from build123d import *

# Parameters (mm, degrees)
SKETCH1_R           = 2.286
BOSS_EXTRUDE1_DEPTH = 12.7
SKETCH5_R           = 2.286
CUT_EXTRUDE3_DEPTH  = 12.7
FILLET1_R           = 4.87
FILLET2_R           = 4.87
SKETCH7_W           = 50.304618045
SKETCH7_H           = 38.1
CUT_EXTRUDE4_DEPTH  = 6.35


with BuildPart() as part:
    # Sketch1 → Boss-Extrude1 (new body)
    with BuildSketch(Plane(origin=(0, 0, 0), x_dir=(1, 0, 0), z_dir=(0, 1, 0))):
        with BuildLine():
            Line((-291.755501553, 191.396492393), (-280.151228022, 178.973093671))
            ThreePointArc((-280.151228022, 178.973093671), (-270.685286175, 182.170263236), (-266.850883508, 191.396492393))
            Line((-266.850883508, 191.396492393), (-254.150883508, 191.396492393))
            Line((-254.150883508, 191.396492393), (-254.150883508, 127.896492393))
            Line((-254.150883508, 127.896492393), (-304.455501553, 127.896492393))
            Line((-304.455501553, 127.896492393), (-304.455501553, 191.396492393))
            Line((-304.455501553, 191.396492393), (-291.755501553, 191.396492393))
        make_face()
        with Locations(Location((-297.746130931, 134.246492393, 0), (0, 0, 270))):
            Circle(SKETCH1_R, mode=Mode.SUBTRACT)
        with Locations(Location((-278.990383135, 134.246492393, 0), (0, 0, 270))):
            Circle(SKETCH1_R, mode=Mode.SUBTRACT)
        with Locations(Location((-260.86025413, 134.246492393, 0), (0, 0, 270))):
            Circle(SKETCH1_R, mode=Mode.SUBTRACT)
    extrude(amount=BOSS_EXTRUDE1_DEPTH)

    # Sketch5 → Cut-Extrude3 (cut)
    with BuildSketch(Plane(origin=(0, 0, -191.396492393), x_dir=(-1, 0, 0), z_dir=(0, 0, -1))):
        with Locations((260.500883508, 6.35)):
            Circle(SKETCH5_R)
        with Locations((298.105501553, 6.35)):
            Circle(SKETCH5_R)
    extrude(amount=-CUT_EXTRUDE3_DEPTH, mode=Mode.SUBTRACT)

    # Fillet1
    fillet1_edges = [part.edges().sort_by_distance(p)[0] for p in [
        (-304.455501553, 6.35, -127.896492393),
    ]]
    fillet(fillet1_edges, radius=FILLET1_R)

    # Fillet2
    fillet2_edges = [part.edges().sort_by_distance(p)[0] for p in [
        (-254.150883508, 6.35, -127.896492393),
    ]]
    fillet(fillet2_edges, radius=FILLET2_R)

    # Sketch7 → Cut-Extrude4 (cut)
    with BuildSketch(Plane(origin=(0, 12.7, 0), x_dir=(1, 0, 0), z_dir=(0, 1, 0))):
        with Locations((-279.303192531, 146.946492393)):
            Rectangle(SKETCH7_W, SKETCH7_H)
    extrude(amount=-CUT_EXTRUDE4_DEPTH, mode=Mode.SUBTRACT)


solid = part.part
The model under review builds one solid part; all positions refer to its coordinate system, in mm. A direction names the side the tool comes from. Round coordinates to 2 decimals unless told otherwise and drop trailing zeros. Write each loop counter-clockwise with the first axis right and the second up, starting at its lowest first coordinate (ties: lowest second). Pieces come first, ordered by that corner, then holes. Notation, with made-up numbers: (-37, -37.5) - (-2, -37.5) arc R26 cw to (-2, -15.5) - close; hole circle Ø7 at (51.5, -11.5). An arc over 180 degrees is marked (long way). One line per item, written item: value. Start each with the question number.
1. Consider section D-D on z = -141.5. Write out the cut boundary in (x, y).
2. To check wall thickness, follow L1, parallel to X at y = 5.75, z = -185.5; L2, parallel to X at y = 1.25, z = -136; L3, parallel to Z at x = -262, y = 1.5. State the ranges of each line that lie inside material, in increasing order. Write a range as from..to.
3. The part is to be moulded in two halves that separate along Y. For faces 5 (the face through (-262.61, 5.47, -185.14)), 6 (the face through (-260, 6, -178.696)), 7 (the face through (-263.1, 3.1, -134.7)), 8 (the face through (-280, 6.35, -147)), say which applies: released by +Y, released by -Y, zero draft, split by the parting line, or undercut.
4. Machinability: for faces 1 (the face through (-286.035, 6.261, -185.272)), 2 (the face through (-300.217, 5.474, -185.135)), 3 (the face through (-303.067, 3.219, -129.361)), 4 (the face through (-280, 10, -165.996)), which of the approach directions +Z, -Z, +X, -X, +Y, -Y give a long, thin tool a straight path to every point of the face, cutting with its end or side? Answer none if there is none.
5. Consider section C-C on y = 9.5. Write out the cut boundary in (x, z), and give its area (3 significant figures).
6. Clearance check with flat-ended pins moving along their axes: P1, Ø11.5, axis at x = -287.5, z = -138.5, coming from the +Y side; P2, Ø1.4, axis at x = -261, y = 6.5, coming from the -Z side. State where each tip first meets the part, or that it passes through.
7. Consider section A-A on y = 5.25. Write out the cut boundary in (x, z), and give its area (3 significant figures).
8. Consider section B-B on x = -294.5. Write out the cut boundary in (y, z).
Checks:
1. outline: (-304.46, 0) - (-254.15, 0) - (-254.15, 6.35) - (-304.46, 6.35) - close
2. L1: x = -304.46..-300.31, -295.9..-286.25, -268.17..-262.71, -258.3..-254.15
2. L2: x = -304.46..-299.21, -296.28..-280.46, -277.52..-262.33, -259.39..-254.15
2. L3: z = -191.4..-136.23, -132.26..-127.9
3. face 5: undercut
3. face 6: undercut
3. face 7: zero draft
3. face 8: released by +Y
4. face 1: -Z, +Y, -Y
4. face 2: -Z
4. face 3: +Z, -X, +Y, -Y
4. face 4: +Z, +X, -X, +Y
5. outline: (-304.46, -191.4) - (-291.76, -191.4) - (-280.15, -178.97) arc R12.1 cw to (-266.85, -191.4) - (-254.15, -191.4) - (-254.15, -166) - (-304.46, -166) - close
5. area: 1,070 mm^2
6. P1: stops at y = 6.35
6. P2: stops at z = -178.7
7. outline: (-304.46, -191.4) - (-300.11, -191.4) - (-300.11, -178.7) - (-296.1, -178.7) - (-296.1, -191.4) - (-291.76, -191.4) - (-280.15, -178.97) arc R12.1 cw to (-266.85, -191.4) - (-262.5, -191.4) - (-262.5, -178.7) - (-258.5, -178.7) - (-258.5, -191.4) - (-254.15, -191.4) - (-254.15, -132.77) arc R4.87 ccw to (-259.02, -127.9) - (-299.59, -127.9) arc R4.87 ccw to (-304.46, -132.77) - close; hole circle Ø4.57 at (-297.75, -134.25); hole circle Ø4.57 at (-278.99, -134.25); hole circle Ø4.57 at (-260.86, -134.25)
7. area: 2,830 mm^2
8. outline: (0, -191.4) - (12.7, -191.4) - (12.7, -166) - (6.35, -166) - (6.35, -127.9) - (0, -127.9) - close
